Model file for the job. Use its own axes, mm. A direction names the side the tool comes from. Coordinates: 2 decimals unless noted, no trailing zeros. Write each loop counter-clockwise with the first axis right and the second up, starting at its lowest first coordinate (ties: lowest second). Pieces come first, ordered by that corner, then holes. Notation, with made-up numbers: M -1,53 L 52,53 A15 cw 52,63 Z; hole C 41,-26 d10. An arc over 180 degrees is marked long. Answer in a Markdown table with one row per item. Add a question column.
```python
from build123d import *

# Parameters (mm, degrees)
SKETCH_1_W          = 196
SKETCH_1_H          = 130
EXTRUDE_1_DEPTH     = 4
SKETCH_3_W          = 196
SKETCH_3_H          = 69
EXTRUDE_2_DEPTH     = 7.5
SKETCH_4_W          = 4
SKETCH_4_H          = 60
EXTRUDE_3_DEPTH     = 33.1
SKETCH_2_R          = 1.7
CUT_EXTRUDE_1_DEPTH = 236.474520915
SKETCH_5_R          = 1.7
CUT_EXTRUDE_2_DEPTH = 236.474520915
FILLET_1_R          = 3
SKETCH_7_R          = 0.6
SKETCH_7_W          = 20
SKETCH_7_H          = 10
CUT_EXTRUDE_3_DEPTH = 236.474520915
SKETCH_8_R          = 1.75
CUT_EXTRUDE_4_DEPTH = 40


with BuildPart() as part:
    # ｽｹｯﾁ1 → ﾎﾞｽ - 押し出し1 (new body)
    with BuildSketch(Plane.XY):
        with Locations((98, 65)):
            Rectangle(SKETCH_1_W, SKETCH_1_H)
    extrude(amount=EXTRUDE_1_DEPTH)

    # ｽｹｯﾁ3 → ﾎﾞｽ - 押し出し2 (add)
    with BuildSketch(Plane(origin=(0, 0, 0), x_dir=(-1, 0, 0), z_dir=(0, 0, -1))):
        with Locations((-98, 34.5)):
            Rectangle(SKETCH_3_W, SKETCH_3_H)
    extrude(amount=EXTRUDE_2_DEPTH)

    # ｽｹｯﾁ4 → ﾎﾞｽ - 押し出し3 (add)
    with BuildSketch(Plane.ZY):
        with Locations((2, 100)):
            Rectangle(SKETCH_4_W, SKETCH_4_H)
    extrude(amount=EXTRUDE_3_DEPTH)

    # ｽｹｯﾁ2 → ｶｯﾄ - 押し出し1 (cut, through all)
    with BuildSketch(Plane.XY.offset(4)):
        with Locations((191, 5)):
            Circle(SKETCH_2_R)
        with Locations((192.5, 126.5)):
            Circle(SKETCH_2_R)
        with Locations((191, 65)):
            Circle(SKETCH_2_R)
        with Locations((6, 5)):
            Circle(SKETCH_2_R)
        with Locations((6, 65)):
            Circle(SKETCH_2_R)
    extrude(amount=-CUT_EXTRUDE_1_DEPTH, mode=Mode.SUBTRACT)

    # ｽｹｯﾁ5 → ｶｯﾄ - 押し出し2 (cut, through all)
    with BuildSketch(Plane.XY.offset(4)):
        with Locations((-29.6, 126.5)):
            Circle(SKETCH_5_R)
        with Locations((-29.6, 73.5)):
            Circle(SKETCH_5_R)
    extrude(amount=-CUT_EXTRUDE_2_DEPTH, mode=Mode.SUBTRACT)

    # ﾌｨﾚｯﾄ1
    fillet_1_edges = [part.edges().sort_by_distance(p)[0] for p in [
        (196, 130, 2),
        (196, 0, -1.75),
    ]]
    fillet(fillet_1_edges, radius=FILLET_1_R)

    # ｽｹｯﾁ7 → ｶｯﾄ - 押し出し3 (cut, through all)
    with BuildSketch(Plane.XY.offset(4)):
        with Locations((174, 41)):
            Circle(SKETCH_7_R)
        with Locations((162, 41)):
            Circle(SKETCH_7_R)
        with Locations((174, 29)):
            Circle(SKETCH_7_R)
        with Locations((162, 29)):
            Circle(SKETCH_7_R)
        with Locations((166, 35)):
            Rectangle(SKETCH_7_W, SKETCH_7_H)
    extrude(amount=-CUT_EXTRUDE_3_DEPTH, mode=Mode.SUBTRACT)

    # ｽｹｯﾁ8 → ｶｯﾄ - 押し出し4 (cut)
    with BuildSketch(Plane.XY.offset(4)):
        with Locations((186, 53.5)):
            Circle(SKETCH_8_R)
        with Locations((153.85, 53.5)):
            Circle(SKETCH_8_R)
        with Locations((153.85, 16.5)):
            Circle(SKETCH_8_R)
        with Locations((186, 16.5)):
            Circle(SKETCH_8_R)
    extrude(amount=-CUT_EXTRUDE_4_DEPTH, mode=Mode.SUBTRACT)


solid = part.part
```
1) Slice it at D-D (y = 46). Give the cut face in (x, z).
2) Flat gauge pins, fed straight in: pin 1 Ø1.2 at (x, z) = (-15, 1.5) entering from -Y; pin 2 Ø4.5 at (x, y) = (192.5, 126.5) entering from -Z; pin 3 Ø1 at (x, y) = (174, 29) entering from -Z; pin 4 Ø5 at (x, z) = (73, -6) entering from +Y. Where does each tip first touch, or does it go through?
3) Drill centre lines: probe 1 along Y at (x, z) = (186, 0.75); probe 2 along X at (y, z) = (41, -2.75); probe 3 along X at (y, z) = (126.5, 1.95). Where is each one in solid material? Low to high.
4) Slice it at B-B (x = 63). Give the cut face in (y, z).
5) Two-plate mould, pull along Y, no slides. Class faces 4 (the face through (156, 35, -2)), 5 (the face through (-16, 70, 2)), 6 (the face through (-33.1, 100, 2)): released by +Y, released by -Y, zero draft, split by the parting line, or undercut.
6) Slice it at C-C (y = 108.5). Give the cut face in (x, z).
7) Slice it at A-A (z = -3.5). Count the separate pieces of the cut face and the enclosed holes in it, then the cut area to 3 significant figures.
8) Which spindle directions (+Z, -Z, +X, -X, +Y, -Y) get a long thin tool onto all of the face, cutting with end or side? Do faces 1 (the face through (0, 35, -2)), 2 (the face through (176, 35, -2)), 3 (the face through (99, 69, -4)). Say none if no direction does.
Ans:
| question | item | result |
|---|---|---|
| 1 | outline | M 0,-7.5 L 196,-7.5 L 196,4 L 0,4 Z |
| 2 | pin 1 | stops at y = 70 |
| 2 | pin 2 | stops at z = 0 |
| 2 | pin 3 | passes through |
| 2 | pin 4 | stops at y = 69 |
| 3 | probe 1 | y = 0 to 14.75, 18.25 to 51.75, 55.25 to 130 |
| 3 | probe 2 | x = 0 to 161.4, 162.6 to 173.4, 174.6 to 196 |
| 3 | probe 3 | x = -33.1 to -31.3, -27.9 to 190.8, 194.2 to 196 |
| 4 | outline | M 0,-7.5 L 69,-7.5 L 69,0 L 130,0 L 130,4 L 0,4 Z |
| 5 | face 4 | undercut |
| 5 | face 5 | released by -Y |
| 5 | face 6 | zero draft |
| 6 | outline | M -33.1,0 L 196,0 L 196,4 L -33.1,4 Z |
| 7 | separate pieces | 1 |
| 7 | enclosed holes | 13 |
| 7 | area | 13,200 mm2 |
| 8 | face 1 | +Z, -Z, -X, -Y |
| 8 | face 2 | +Z, -Z |
| 8 | face 3 | -Z, +X, -X, +Y |
